Build history of the part. All positions in model axes, mm. A direction names the side the tool comes from. Round coordinates to 2 decimals unless told otherwise and drop trailing zeros. Write each loop counter-clockwise with the first axis right and the second up, starting at its lowest first coordinate (ties: lowest second). Pieces come first, ordered by that corner, then holes. Notation, with made-up numbers: (63, 25) -> (69, 25) arc R14 ccw to (69, 41) -> close; hole circle Ø7 at (-27.5, 30). An arc over 180 degrees is marked (long way). Answer as CSV lines item,"result".
from build123d import *

# Parameters (mm, degrees)
F0_R     = 2.15265
F0_R_2   = 3.96875
F0_R_3   = 7.9375
F0_R_4   = 1.7272
F1_DEPTH = 3.175
F2_R     = 4.7625
F4_DEPTH = 3.175


with BuildPart() as f1:
    # F0 (on Top) → F1 (new body)
    with BuildSketch(Plane.XY):
        with BuildLine():
            Line((21.1458048519, 50.3316372454), (-14.5929161967, 14.5929161967))
            ThreePointArc((-14.5929161967, 14.5929161967), (-20.6375, 0), (-14.5929161967, -14.5929161967))
            Line((-14.5929161967, -14.5929161967), (21.1458048519, -50.3316372454))
            ThreePointArc((21.1458048519, -50.3316372454), (22.6908710507, -51.3640174736), (24.5134008973, -51.7265412))
            Line((24.5134008973, -51.7265412), (84.9529040973, -51.7265412))
            Line((84.9529040973, -51.7265412), (84.9529040973, 51.7265412))
            Line((84.9529040973, 51.7265412), (24.5134008973, 51.7265412))
            ThreePointArc((24.5134008973, 51.7265412), (22.6908710507, 51.3640174736), (21.1458048519, 50.3316372454))
        make_face()
        with Locations((24.5134008973, -46.9640412)):
            Circle(F0_R, mode=Mode.SUBTRACT)
        with Locations((-10.6640541438, -10.6640541438)):
            Circle(F0_R_2, mode=Mode.SUBTRACT)
        Circle(F0_R_3, mode=Mode.SUBTRACT)
        with Locations((10.6640541438, -10.6640541438)):
            Circle(F0_R_4, mode=Mode.SUBTRACT)
        with Locations((80.1904040973, -46.9640412)):
            Circle(F0_R, mode=Mode.SUBTRACT)
        with Locations((-10.6640541438, 10.6640541438)):
            Circle(F0_R_4, mode=Mode.SUBTRACT)
        with Locations((10.6640541438, 10.6640541438)):
            Circle(F0_R_2, mode=Mode.SUBTRACT)
        with Locations((24.5134008973, 46.9640412)):
            Circle(F0_R, mode=Mode.SUBTRACT)
        with Locations((34.0384008973, 5.55625)):
            Circle(F0_R_4, mode=Mode.SUBTRACT)
        with Locations((70.6654040973, 5.55625)):
            Circle(F0_R_4, mode=Mode.SUBTRACT)
        with Locations((70.6654040973, 46.9640412)):
            Circle(F0_R_4, mode=Mode.SUBTRACT)
        with Locations((80.1904040973, 46.9640412)):
            Circle(F0_R, mode=Mode.SUBTRACT)
    extrude(amount=F1_DEPTH)

    # F2
    f2_edges = [f1.edges().sort_by_distance(p)[0] for p in [
        (84.952904, 51.726541, 1.5875),
        (84.952904, -51.726541, 1.5875),
    ]]
    fillet(f2_edges, radius=F2_R)

    # F3 (on face) → F4 (cut, through all)
    with BuildSketch(Plane.XY.offset(3.175)):
        with BuildLine():
            Line((52.0652126973, -37.68725), (84.9529040973, -37.68725))
            Line((84.9529040973, -37.68725), (84.9529040973, -0.22225))
            Line((84.9529040973, -0.22225), (52.0652126973, -0.22225))
            ThreePointArc((52.0652126973, -0.22225), (33.3327126973, -18.95475), (52.0652126973, -37.68725))
        make_face()
    extrude(amount=-F4_DEPTH, mode=Mode.SUBTRACT)


solid = f1.part
1. Probe line 1 along Y through (x, z) = (61.5, 1.85); line 2 along X through (y, z) = (10.5, 0.25); line 3 along Y through (x, z) = (-10, 0.9). List the from-to ranges inside material, lowest first.
Results found:
line 1,"y = -51.73 to -37.69, -0.22 to 51.73"
line 2,"x = -17.77 to -12.38, -8.94 to 6.7, 14.63 to 84.95"
line 3,"y = -19.19 to -14.58, -6.75 to 9.07, 12.26 to 19.19"
2. Mould opens along Y. For faces 1 (the cylindrical face through (22.667, -51.354, 1.565)), 2 (the cylindrical face through (24.23, -44.83, 1.57)), 3 (the cylindrical face through (83.52, 50.37, 1.61)), 4 (the flat face through (84.953, -42, 2)) say: +Y half, -Y half, draft (parallel to the pull), parting line (faces both ways), or undercut.
Results found:
face 1,"-Y half"
face 2,"undercut"
face 3,"+Y half"
face 4,"draft"
3. Drop flat-ended pins along their axis: pin 1 Ø3 at (x, y) = (-10.66, 10.66) entering from -Z; pin 2 Ø4.5 at (x, y) = (10.66, -10.66) entering from +Z (3 decimals). Give the stop position or say it passes through.
Results found:
pin 1,"passes through"
pin 2,"stops at z = 3.175"
4. Which spindle directions (+Z, -Z, +X, -X, +Y, -Y) get a long thin tool onto all of the face, cutting with end or side? Do faces 5 (the flat face through (69, -0.222, 2)), 6 (the cylindrical face through (82.244, 47.611, 1.565)). Say none if no direction does.
Results found:
face 5,"+Z, -Z, +X"
face 6,"+Z, -Z"
5. Cut at D-D, the plane y = 30.5. Write the cut outline in (x, z) (3 decimals).
Results found:
outline,"(1.314, 0) -> (84.953, 0) -> (84.953, 3.175) -> (1.314, 3.175) -> close"
6. Cut at A-A, the plane x = 0. Write the cut outline in (y, z) (1 decimal).
Results found:
outline,"(-29.2, 0) -> (-7.9, 0) -> (-7.9, 3.2) -> (-29.2, 3.2) -> close; (7.9, 0) -> (29.2, 0) -> (29.2, 3.2) -> (7.9, 3.2) -> close"
7. Cut at B-B, the plane z = 0.7. Count the separate pieces of the cut face and the enclosed holes in it, then the cut area to 3 significant figures.
Results found:
separate pieces,"1"
enclosed holes,"12"
area,"6,840 mm2"
8. Cut at C-C, the plane y = -35.5. Write the cut outline in (x, z) (3 decimals).
Results found:
outline,"(6.314, 0) -> (43.281, 0) -> (43.281, 3.175) -> (6.314, 3.175) -> close"
